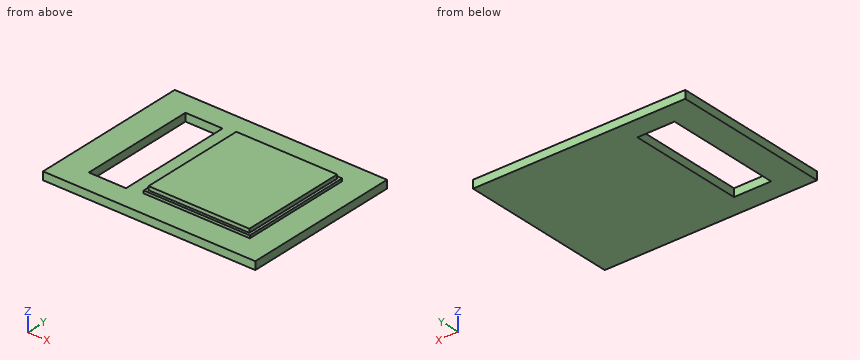
from build123d import *

# Parameters (mm, degrees)
SKETCH1_W           = 40
SKETCH1_H           = 30
BOSS_EXTRUDE1_DEPTH = 1.5
SKETCH2_W           = 20
SKETCH2_H           = 21
BOSS_EXTRUDE2_DEPTH = 0.5
SKETCH4_W           = 19
SKETCH4_H           = 20
BOSS_EXTRUDE3_DEPTH = 0.7
SKETCH5_W           = 7
SKETCH5_H           = 22
CUT_EXTRUDE1_DEPTH  = 1.5


with BuildPart() as part:
    # Sketch1 → Boss-Extrude1 (new body)
    with BuildSketch(Plane.XY):
        Rectangle(SKETCH1_W, SKETCH1_H)
    extrude(amount=BOSS_EXTRUDE1_DEPTH)

    # Sketch2 → Boss-Extrude2 (add)
    with BuildSketch(Plane.XY.offset(1.5)):
        with Locations((5.25, 0)):
            Rectangle(SKETCH2_W, SKETCH2_H)
    extrude(amount=BOSS_EXTRUDE2_DEPTH)

    # Sketch4 → Boss-Extrude3 (add)
    with BuildSketch(Plane.XY.offset(2)):
        with Locations((5.25, 0)):
            Rectangle(SKETCH4_W, SKETCH4_H)
    extrude(amount=BOSS_EXTRUDE3_DEPTH)

    # Sketch5 → Cut-Extrude1 (cut)
    with BuildSketch(Plane.XY.offset(1.5)):
        with Locations((-11.166666, 0)):
            Rectangle(SKETCH5_W, SKETCH5_H)
    extrude(amount=-CUT_EXTRUDE1_DEPTH, mode=Mode.SUBTRACT)


solid = part.part
Geometry check sheet. Reference: the model listing, model coordinates, mm. Coordinates: 2 decimals unless noted, no trailing zeros. Order: outer loops, then holes, each group sorted by start corner. A loop starts at its lowest first (then second) coordinate and runs counter-clockwise, first axis right, second up. Notation, with made-up numbers: (27, 60.5) - (65, 60.5) arc R17 ccw to (65, 86.5) - close; hole circle Ø11 at (-30.75, -6). An arc over 180 degrees is marked (long way). Answer in a Markdown table with one row per item. Add a question column.
1) Material ranges on line 1 along Y through (x, z) = (-8, 0.6); line 2 along X through (y, z) = (-8.75, 0.3); line 3 along Y through (x, z) = (1, 2.2), recorded low to high. Write a range as [from, to].
2) Cross-section at C-C, the plane x = -12. Record the cut outline in (y, z), then the cut area to 3 significant figures.
3) Cross-section at A-A, the plane y = 2.25. Record the cut outline in (x, z).
4) Gauge pin test, flat ends, axial feed: P1, Ø0.8, axis at y = 0.5, z = 2, coming from the -X side; P2, Ø0.6, axis at y = -1.5, z = 2, coming from the +X side; P3, Ø10, axis at x = -14.5, y = 5, coming from the +Z side. Record the tip position at first contact, or that the pin passes through.
5) Cross-section at B-B, the plane z = 0.6. Record the cut outline in (x, y).
6) Cross-section at D-D, the plane x = 3. Record the cut outline in (y, z), then the cut area to 3 significant figures.
Check result:
| question | item | result |
|---|---|---|
| 1 | line 1 | y = [-15, -11], [11, 15] |
| 1 | line 2 | x = [-20, -14.67], [-7.67, 20] |
| 1 | line 3 | y = [-10, 10] |
| 2 | outline | (-15, 0) - (-11, 0) - (-11, 1.5) - (-15, 1.5) - close; (11, 0) - (15, 0) - (15, 1.5) - (11, 1.5) - close |
| 2 | area | 12.0 mm² |
| 3 | outline | (-20, 0) - (-14.67, 0) - (-14.67, 1.5) - (-20, 1.5) - close; (-7.67, 0) - (20, 0) - (20, 1.5) - (15.25, 1.5) - (15.25, 2) - (14.75, 2) - (14.75, 2.7) - (-4.25, 2.7) - (-4.25, 2) - (-4.75, 2) - (-4.75, 1.5) - (-7.67, 1.5) - close |
| 4 | P1 | stops at x = -4.75 |
| 4 | P2 | stops at x = 15.25 |
| 4 | P3 | stops at z = 1.5 |
| 5 | outline | (-20, -15) - (20, -15) - (20, 15) - (-20, 15) - close; hole (-14.67, -11) - (-7.67, -11) - (-7.67, 11) - (-14.67, 11) - close |
| 6 | outline | (-15, 0) - (15, 0) - (15, 1.5) - (10.5, 1.5) - (10.5, 2) - (10, 2) - (10, 2.7) - (-10, 2.7) - (-10, 2) - (-10.5, 2) - (-10.5, 1.5) - (-15, 1.5) - close |
| 6 | area | 69.5 mm² |
